Could you check a few things on this model? Use its own coordinates, in mm. Face numbers are marked on the shaded views. A direction names the side the tool comes from. Give positions to 0.01 mm unless a question says otherwise; leave off trailing zeros. Loops run counter-clockwise (first coordinate to the right, second up) from the corner with the lowest first, then second, coordinate; pieces in that order, holes last. Notation, with made-up numbers: M -11,48 L 18,48 A10 cw 18,66 Z; hole C 33.5,43.25 d6. An arc over 180 degrees is marked long. Answer in a Markdown table with one row per item. Add a question column.
1. If we section it at C-C on y = -45.5: List the corners of the cut face in (x, z) for me (3 decimals).
2. I need wall thicknesses on line 1 along X through (y, z) = (-42, -18); line 2 along Z through (x, y) = (-3, -21). Which ranges of each line are inside material? Lowest first, please. Write a range as from..to.
3. If we section it at B-B on z = -29: List the corners of the cut face in (x, y) for me.
4. Which directions (+Z, -Z, +X, -X, +Y, -Y) give clear straight access to the entire face, cutting with the end or side of a thin tool? Please do the marked faces 1, 2, 3 and 4.
5. I'm going to push flat-ended pins straight in: pin 1 Ø5 at (x, z) = (-5.5, -22) entering from +Y; pin 2 Ø1.3 at (x, z) = (-1.5, 0.5) entering from -Y (3 decimals); pin 3 Ø2 at (x, y) = (-27, -16) entering from -Z; pin 4 Ø0.8 at (y, z) = (-86, -1) entering from +X. Where does each tip first touch, or does it pass through?
6. If we section it at A-A on y = -31: List the corners of the cut face in (x, z) for me (3 decimals).
7. If we section it at D-D on x = -20.5: List the corners of the cut face in (y, z) for me.
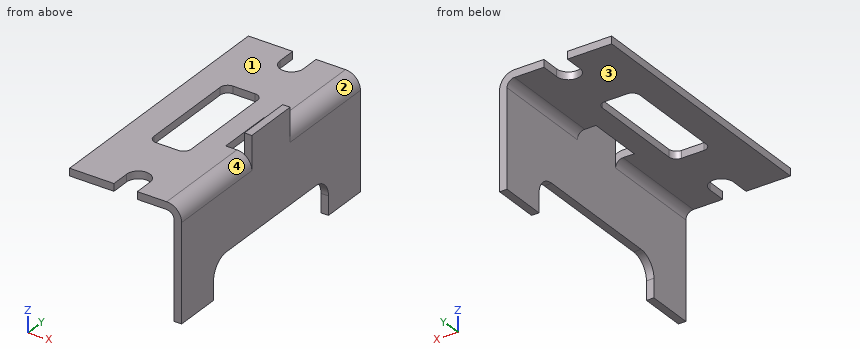
```python
from build123d import *

# Parameters (mm, degrees)
F1_DEPTH      = 88.9
F2_W          = 2.54
F2_H          = 19.05
F2_W_2        = 3.81
F3_DEPTH      = 25.4
F4_W          = 2.54
F4_H          = 19.05
F5_DEPTH      = 6.35
F5_DEPTH_BACK = 6.35
F7_DEPTH      = 25.4
F9_DEPTH      = 25.4
F11_DEPTH     = 25.4


with BuildPart() as f1:
    # F0 (on Front) → F1 (new body)
    with BuildSketch(Plane.XZ):
        with BuildLine():
            ThreePointArc((0, -5.08), (-1.4878975516, -1.4878975516), (-5.08, 0))
            Line((-5.08, 0), (-38.1, 0))
            Line((-38.1, 0), (-38.1, -2.54))
            Line((-38.1, -2.54), (-5.08, -2.54))
            ThreePointArc((-5.08, -2.54), (-3.2839487758, -3.2839487758), (-2.54, -5.08))
            Line((-2.54, -5.08), (-2.54, -38.1))
            Line((-2.54, -38.1), (0, -38.1))
            Line((0, -38.1), (0, -5.08))
        make_face()
    extrude(amount=F1_DEPTH)

    # F2 (on face) → F3 (cut)
    with BuildSketch(Plane.XY):
        with Locations((-3.81, -44.45)):
            Rectangle(F2_W, F2_H)
        with Locations((-6.985, -44.45)):
            Rectangle(F2_W_2, F2_H)
    extrude(amount=-F3_DEPTH, mode=Mode.SUBTRACT)

    # F4 (on face) → F5 (join, two sides)
    with BuildSketch(Plane.XY) as f5_sk:
        with Locations((-1.27, -44.45)):
            Rectangle(F4_W, F4_H)
    extrude(amount=F5_DEPTH)
    extrude(f5_sk.sketch, amount=-F5_DEPTH_BACK)

    # F6 (on face) → F7 (cut)
    with BuildSketch(Plane.XY):
        with BuildLine():
            Line((-23.01875, 0), (-23.01875, -6.35))
            ThreePointArc((-23.01875, -6.35), (-19.05, -10.31875), (-15.08125, -6.35))
            Line((-15.08125, -6.35), (-15.08125, 0))
            Line((-15.08125, 0), (-23.01875, 0))
        make_face()
        with BuildLine():
            Line((-15.08125, -88.9956355095), (-15.08125, -82.55))
            ThreePointArc((-15.08125, -82.55), (-19.05, -78.58125), (-23.01875, -82.55))
            Line((-23.01875, -82.55), (-23.01875, -88.9956355095))
            Line((-23.01875, -88.9956355095), (-15.08125, -88.9956355095))
        make_face()
    extrude(amount=-F7_DEPTH, mode=Mode.SUBTRACT)

    # F8 (on face) → F9 (cut)
    with BuildSketch(Plane.XY):
        with BuildLine():
            Line((-18.415, -25.4), (-26.035, -25.4))
            ThreePointArc((-26.035, -25.4), (-27.8310512242, -26.1439487758), (-28.575, -27.94))
            Line((-28.575, -27.94), (-28.575, -60.96))
            ThreePointArc((-28.575, -60.96), (-27.8310512242, -62.7560512242), (-26.035, -63.5))
            Line((-26.035, -63.5), (-18.415, -63.5))
            ThreePointArc((-18.415, -63.5), (-16.6189487758, -62.7560512242), (-15.875, -60.96))
            Line((-15.875, -60.96), (-15.875, -27.94))
            ThreePointArc((-15.875, -27.94), (-16.6189487758, -26.1439487758), (-18.415, -25.4))
        make_face()
    extrude(amount=-F9_DEPTH, mode=Mode.SUBTRACT)

    # F10 (on face) → F11 (cut)
    with BuildSketch(Plane.YZ):
        with BuildLine():
            Line((-73.025, -31.75), (-73.025, -38.1))
            Line((-73.025, -38.1), (-15.875, -38.1))
            Line((-15.875, -38.1), (-15.875, -31.75))
            ThreePointArc((-15.875, -31.75), (-17.7348719395, -27.2598719395), (-22.225, -25.4))
            Line((-22.225, -25.4), (-66.675, -25.4))
            ThreePointArc((-66.675, -25.4), (-71.1651280605, -27.2598719395), (-73.025, -31.75))
        make_face()
    extrude(amount=-F11_DEPTH, mode=Mode.SUBTRACT)


solid = f1.part
```
Results:
| question | item | result |
|---|---|---|
| 1 | outline | M -38.1,-2.54 L -28.575,-2.54 L -28.575,0 L -38.1,0 Z; M -15.875,-2.54 L -8.89,-2.54 L -8.89,0 L -15.875,0 Z; M -2.54,-25.4 L 0,-25.4 L 0,6.35 L -2.54,6.35 Z |
| 2 | line 1 | -2.54..0 |
| 2 | line 2 | -3.62..-0.45 |
| 3 | outline | M -2.54,-88.9 L 0,-88.9 L 0,-72.4 L -2.54,-72.4 Z; M -2.54,-16.5 L 0,-16.5 L 0,0 L -2.54,0 Z |
| 4 | face 1 | +Z, -X, +Y, -Y |
| 4 | face 2 | +Z, +X, +Y |
| 4 | face 3 | -Z, -X, +Y, -Y |
| 4 | face 4 | +Z, +X, -Y |
| 5 | pin 1 | through |
| 5 | pin 2 | y = -53.975 |
| 5 | pin 3 | z = -2.54 |
| 5 | pin 4 | x = -1.58 |
| 6 | outline | M -38.1,-2.54 L -28.575,-2.54 L -28.575,0 L -38.1,0 Z; M -15.875,-2.54 L -5.08,-2.54 A2.54 cw -2.54,-5.08 L -2.54,-25.4 L 0,-25.4 L 0,-5.08 A5.08 ccw -5.08,0 L -15.875,0 Z |
| 7 | outline | M -78.86,-2.54 L -63.5,-2.54 L -63.5,0 L -78.86,0 Z; M -25.4,-2.54 L -10.04,-2.54 L -10.04,0 L -25.4,0 Z |
